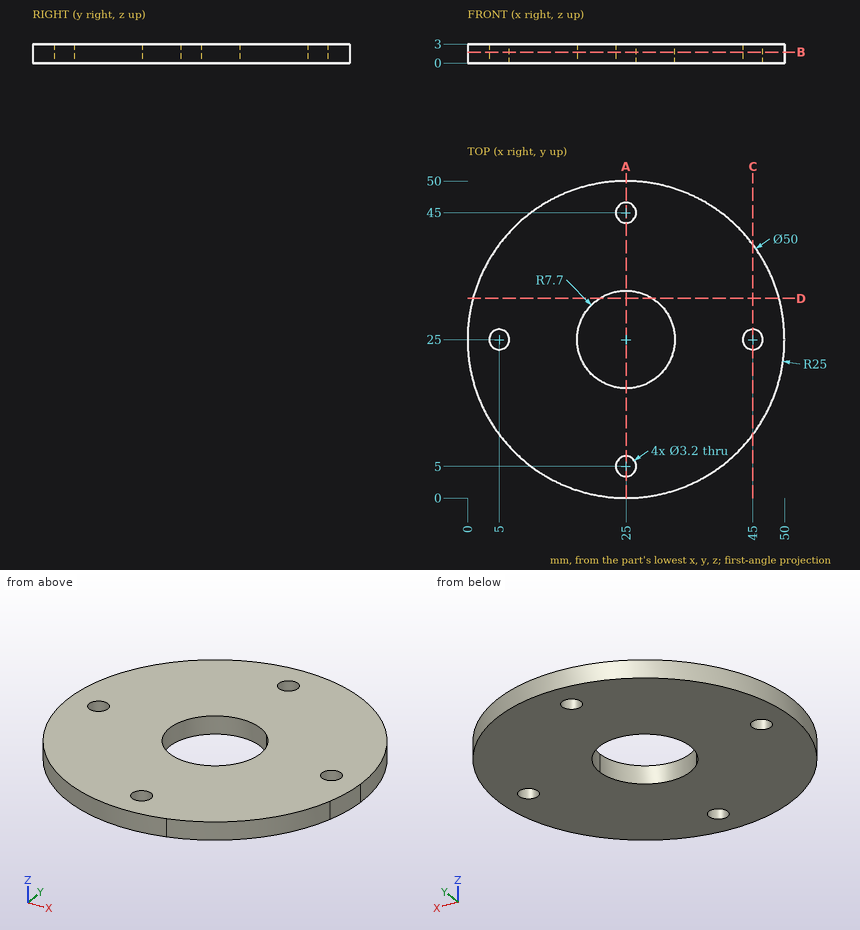
The drawing under review shows one solid part. Ordinate dimensions are in mm from its lowest x, y, z. Give positions to 0.01 mm unless a question says otherwise; leave off trailing zeros. Order: outer loops, then holes, each group sorted by start corner. A loop starts at its lowest first (then second) coordinate and runs counter-clockwise, first axis right, second up. Notation, with made-up numbers: (24.25, 61) -> (40.25, 61) arc R20 cw to (40.25, 68) -> close; hole circle Ø3 at (26.5, -5). An arc over 180 degrees is marked (long way). Write item = value, one per line. Start each with the question number.
(1) To check wall thickness, follow line 1 along Y through (x, z) = (25, 2.1); line 2 along X through (y, z) = (29, 2.3). State the ranges of each line that lie inside material, in increasing order.
(2) We need section B-B on z = 1.7. Write out the cut boundary in (x, y).
(3) We need section D-D on y = 31.5. Write out the cut boundary in (x, z), plus the area to 3 significant figures.
(4) For pin 1 (1.9 mm diameter, centred on x = 25, y = 5, fed in from -Z), flat-tipped, find the tip position at first contact; note if it passes through.
(5) We need section C-C on x = 45. Write out the cut boundary in (y, z), plus the area to 3 significant figures.
(6) We need section A-A on x = 25. Write out the cut boundary in (y, z), plus the area to 3 significant figures.
Numbers:
q1.line_1 = 0 to 3.4, 6.6 to 17.3, 32.7 to 43.4, 46.6 to 50
q1.line_2 = 0.32 to 18.42, 31.58 to 49.68
q2.outline = (31.85, 0.96) arc R25 ccw to (49.04, 18.15) arc R25 ccw to (50, 25) arc R25 ccw (long way) to start; hole circle Ø3.2 at (5, 25); hole circle Ø3.2 at (25, 5); hole circle Ø3.2 at (25, 45); hole (30.44, 30.44) arc R7.7 ccw (long way) to (32.7, 25) arc R7.7 ccw to start; hole circle Ø3.2 at (45, 25)
q3.outline = (0.86, 0) -> (20.87, 0) -> (20.87, 3) -> (0.86, 3) -> close; (29.13, 0) -> (49.14, 0) -> (49.14, 3) -> (29.13, 3) -> close
q3.area = 120 mm^2
q4.pin_1 = through
q5.outline = (10, 0) -> (23.4, 0) -> (23.4, 3) -> (10, 3) -> close; (26.6, 0) -> (40, 0) -> (40, 3) -> (26.6, 3) -> close
q5.area = 80.4 mm^2
q6.outline = (0, 0) -> (3.4, 0) -> (3.4, 3) -> (0, 3) -> close; (6.6, 0) -> (17.3, 0) -> (17.3, 3) -> (6.6, 3) -> close; (32.7, 0) -> (43.4, 0) -> (43.4, 3) -> (32.7, 3) -> close; (46.6, 0) -> (50, 0) -> (50, 3) -> (46.6, 3) -> close
q6.area = 84.6 mm^2
